The listing builds one solid part. Answer for the finished solid, in the listing's coordinates (mm). Round coordinates to 2 decimals unless told otherwise and drop trailing zeros. Write each loop counter-clockwise with the first axis right and the second up, starting at its lowest first coordinate (ties: lowest second). Pieces come first, ordered by that corner, then holes. Notation, with made-up numbers: M 33.25,36 L 69.25,36 A29 ccw 69.25,68 Z; hole C 52,11 d2. An arc over 180 degrees is marked long. One line per item, written item: value. Start each with the question number.
(1) Section A-A (x = 162) is taken. Determine the outline of the cut face in (y, z).
(2) Section C-C (z = 5.75) is taken. Determine the outline of the cut face in (x, y), plus the area to 3 significant figures.
(3) Consider probe 1 along Y at (x, z) = (188, 8.75); probe 2 along X at (y, z) = (11, 0.5); probe 3 along X at (y, z) = (-7, 2.25). Determine where each line is inside the solid, lowest interval first.
(4) Section D-D (y = -44.5) is taken. Determine the outline of the cut face in (x, z), plus the area to 3 significant figures.
(5) Section B-B (y = 9.8) is taken. Determine the outline of the cut face in (x, z).
(6) Given P1, Ø6, axis at y = -74.5, z = 9, coming from the +X side; P2, Ø2, axis at x = 154.5, z = 10, coming from the -Y side; P3, Ø7, axis at x = 5, z = 6.5, coming from the +Y side; P4, Ø5.5, axis at x = 162, y = 9.8, coming from the -Z side, each flat-ended and moving along its own axis, determine where each tip first touches the part or whether it passes through.
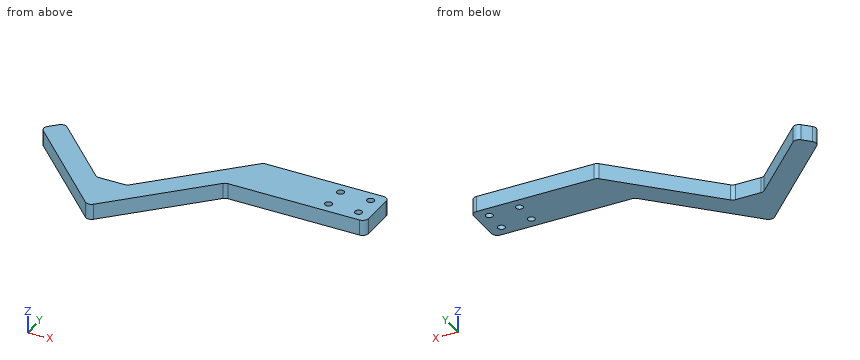
```python
from build123d import *

# Parameters (mm, degrees)
SKETCH1_R           = 3.1
BOSS_EXTRUDE1_DEPTH = 13.5
FILLET1_R           = 5


with BuildPart() as part:
    # Sketch1 → Boss-Extrude1 (new body)
    with BuildSketch(Plane.XY):
        Polygon((13.129942315, -57.580735804), (-13.129942315, -57.580735804), (0, -70.710678119), align=None)
        Polygon((0, -70.710678119), (90.210678119, 19.5), (199, 19.5), (199, -19.5), (78.080735804, -19.5), (0, -97.580735804), (-84.145706961, -13.435028843), (-70.710678119, 0), align=None)
        with Locations((188, -9.8)):
            Circle(SKETCH1_R, mode=Mode.SUBTRACT)
        with Locations((162, -9.8)):
            Circle(SKETCH1_R, mode=Mode.SUBTRACT)
        with Locations((162, 9.8)):
            Circle(SKETCH1_R, mode=Mode.SUBTRACT)
        with Locations((188, 9.8)):
            Circle(SKETCH1_R, mode=Mode.SUBTRACT)
    extrude(amount=BOSS_EXTRUDE1_DEPTH)

    # Fillet1
    fillet1_edges = [part.edges().sort_by_distance(p)[0] for p in [
        (13.129942315, -57.580735804, 6.75),
        (90.210678119, 19.5, 6.75),
        (199, 19.5, 6.75),
        (199, -19.5, 6.75),
        (78.080735804, -19.5, 6.75),
        (0, -97.580735804, 6.75),
        (-84.145706961, -13.435028843, 6.75),
        (-70.710678119, 0, 6.75),
        (-13.129942315, -57.580735804, 6.75),
    ]]
    fillet(fillet1_edges, radius=FILLET1_R)


solid = part.part
```
Recorded:
1. outline: M -19.5,0 L -12.9,0 L -12.9,13.5 L -19.5,13.5 Z; M -6.7,0 L 6.7,0 L 6.7,13.5 L -6.7,13.5 Z; M 12.9,0 L 19.5,0 L 19.5,13.5 L 12.9,13.5 Z
2. outline: M -80.61,-16.97 L -3.54,-94.05 A5 ccw 3.54,-94.05 L 76.62,-20.96 A5 cw 80.15,-19.5 L 194,-19.5 A5 ccw 199,-14.5 L 199,14.5 A5 ccw 194,19.5 L 92.28,19.5 A5 ccw 88.75,18.04 L 14.59,-56.12 A5 cw 11.06,-57.58 L -11.06,-57.58 A5 cw -14.59,-56.12 L -67.18,-3.54 A5 ccw -74.25,-3.54 L -80.61,-9.9 A5 ccw Z; hole C 162,-9.8 d6.2; hole C 162,9.8 d6.2; hole C 188,-9.8 d6.2; hole C 188,9.8 d6.2
2. area: 8,850 mm2
3. probe 1: y = -19.5 to -12.9, -6.7 to 6.7, 12.9 to 19.5
3. probe 2: x = 81.71 to 159.14, 164.86 to 185.14, 190.86 to 199
3. probe 3: x = -77.71 to -63.71, 63.71 to 160.67, 163.33 to 186.67, 189.33 to 199
4. outline: M -53.08,0 L -26.21,0 L -26.21,13.5 L -53.08,13.5 Z; M 26.21,0 L 53.08,0 L 53.08,13.5 L 26.21,13.5 Z
4. area: 725 mm2
5. outline: M 80.51,0 L 158.9,0 L 158.9,13.5 L 80.51,13.5 Z; M 165.1,0 L 184.9,0 L 184.9,13.5 L 165.1,13.5 Z; M 191.1,0 L 199,0 L 199,13.5 L 191.1,13.5 Z
6. P1: stops at x = 26.08
6. P2: stops at y = -19.5
6. P3: stops at y = -57.58
6. P4: passes through
